Autodesk Inventor part; units mm, degrees
ref_plane "Work Plane1" through (0, 0, 0) normal (0, -1, 0) x (1, 0, 0)
ref_plane "YZ Plane" through (0, 0, 0) normal (1, 0, 0) x (0, 1, 0)
ref_plane "XZ Plane" through (0, 0, 0) normal (0, 1, 0) x (-1, 0, 0)
sketch "Sketch1" plane through (0, 0, 0) normal (0, 1, 0) x (-1, 0, 0)
  line L0 (0, 0) -> (27, 0)
  line L1 (27, 0) -> (27, -24)
  line L2 (27, -24) -> (0, -24)
  line L3 (0, -24) -> (0, 0)
  dimension "d0" = 27
  dimension "d1" = 24
extrude "Extrusion1" add sketch "Sketch1" along normal blind 8
sketch "Sketch2" plane through (0, 0, -24) normal (0, 0, -1) x (-1, 0, 0)
  line L0 (0, 0) -> (27, 0)
  line L1 (0, 0) -> (46.1678, 13.2384)
  line L2 (0, 0) -> (48.0283, 0) construction
  line L3 (0, 8) -> (27, 8)
  line L4 (27, 0) -> (27, 8)
  line L5 (0, 8) -> (27, 8)
  line L6 (27, 8) -> (27, 0)
  line L7 (27, 0) -> (0, 0)
  line L8 (0, 0) -> (0, 8)
  point P0 (27, 7.7421)
  dimension "d4" = 16
extrude "Extrusion2" cut sketch "Sketch2" against normal blind 30 contours L1 L4 L0
ref_plane "Work Plane1" through (0, 0, 0) normal (0, -1, 0) x (1, 0, 0)
sketch "Sketch3" plane through (0, 0, 0) normal (0, -1, 0) x (1, 0, 0)
  line L0 (0, 0) -> (0, -24)
  line L1 (0, -12) -> (-4, -12)
  circle A0 centre (-4, -12) radius 2.85
  line L2 (-4, -12) -> (-20, -12)
  line L3 (-12, -12) -> (-12, -20)
  line L4 (-12, -20) -> (-12, -4)
  circle A1 centre (-12, -20) radius 2.85
  circle A2 centre (-20, -12) radius 2.85
  circle A3 centre (-12, -4) radius 2.85
  dimension "d8" = 4
  dimension "d9" = 5.7
  dimension "d10" = 16
  dimension "d11" = 8
  dimension "d12" = 16
  dimension "d13" = 5.7
  dimension "d14" = 5.7
  dimension "d15" = 5.7
extrude "Extrusion3" add sketch "Sketch3" against normal blind 8
sketch "Sketch4" plane through (-4, 0, -12) normal (0, -1, 0) x (1, 0, 0)
  line L0 (4, 12) -> (4, -12)
  line L1 (4, -12) -> (-23.2805, -12)
  line L2 (-23.2805, -12) -> (-23.2805, 12)
  line L3 (-23.2805, 12) -> (4, 12)
  line L4 (4, 12) -> (4, -12)
extrude "Extrusion4" cut sketch "Sketch4" against normal blind 0.5
sketch "Sketch5" plane through (0, 8, 0) normal (0, 1, 0) x (1, 0, 0)
  line L0 (0, 0) -> (0, 24)
  line L1 (-27, 24) -> (-27, 0)
  line L2 (0, 0) -> (-27, 0)
  line L3 (-27, 0) -> (-27, 24)
  line L4 (-27, 24) -> (0, 24)
  line L5 (0, 24) -> (0, 0)
  circle A0 centre (-12, 4) radius 2.85
  circle A1 centre (-12, 20) radius 2.85
  line L6 (-12, 4) -> (-12, 20)
  arc A2 (-1.7437, 13.7412) -> (-1.7437, 10.2588) centre (-4, 12) ccw
  circle A3 centre (-20, 12) radius 2.85
  line L7 (-4, 12) -> (-20, 12)
  circle A4 centre (-12, 12) radius 1.65
  dimension "d20" = 3.3
extrude "Extrusion5" cut sketch "Sketch5" against normal blind 30 contours A4 L7 L6 | L6 L7 A4 | L7 A4 L6 | L6 A4 L7
sketch "Sketch6" plane through (0, 8, 0) normal (0, 1, 0) x (1, 0, 0)
  circle A0 centre (-12, 12) radius 1.65
  circle A1 centre (-12, 12) radius 2.9
  point P0 (0, 0)
  dimension "d23" = 5.8
extrude "Extrusion6" cut sketch "Sketch6" against normal blind 2
sketch "Sketch7" plane through (0, 8, 0) normal (0, 1, 0) x (1, 0, 0)
  line L0 (0, 24) -> (-27, 24)
  line L1 (0, 0) -> (-27, 0)
  line L2 (-27, 0) -> (-27, 24)
  line L3 (-27, 24) -> (0, 24)
  line L4 (0, 24) -> (0, 0)
  circle A0 centre (-12, 12) radius 1.65
  circle A1 centre (-12, 12) radius 2.9
extrude "Extrusion7" add sketch "Sketch7" along normal blind 4 contours L4 L1 L2 L0
sketch "Sketch8" plane through (0, 12, 0) normal (0, 1, 0) x (1, 0, 0)
  circle A0 centre (-12, 12) radius 2.9
  line L0 (-12, 12) -> (-12, -7.1279)
  line L1 (-27, 0) -> (0, 0)
  line L2 (-12, 12) -> (3.3617, 12)
  line L3 (3.3617, 12) -> (3.3617, -5.9927)
  line L4 (3.3617, -5.9927) -> (-12, -5.9927)
  line L5 (-12, -5.9927) -> (-12, 12)
  line L6 (-12, 12) -> (-14, 12)
  line L7 (-14, 12) -> (-14, -1.5388)
  line L8 (-12, 12) -> (-12, 14)
  line L9 (-12, 14) -> (5.1891, 14)
  line L10 (-14, -1.5388) -> (5.1891, -1.5388)
  line L11 (5.1891, -1.5388) -> (5.1891, 14)
  line L12 (5.1891, 14) -> (-14, 14)
  line L13 (-14, 14) -> (-14, -1.5388)
  point P0 (-14, 9.9)
  point P1 (-14, 0)
  point P2 (-12, 0)
  point P3 (-12, -1.5388)
  point P4 (-9.9, 14)
  dimension "d28" = 2
  dimension "d29" = 2
extrude "Extrusion8" cut sketch "Sketch8" against normal blind 4 contours L2 L3 L10 L0 A0 | A0 L9 L11 L10 L3 L2 | L0 L1 L7 A0
sketch "Sketch10" plane through (0, 12, 0) normal (0, 1, 0) x (1, 0, 0)
  line L0 (0, 14) -> (0, 0)
  line L1 (-27, 24) -> (-27, 0)
  line L2 (0, 0) -> (-27, 0)
  line L3 (-27, 0) -> (-27, 24)
  line L4 (-27, 24) -> (0, 24)
  line L5 (0, 24) -> (0, 0)
extrude "Extrusion10" cut sketch "Sketch10" against normal blind 4
sketch "Sketch11" plane through (0, 8, 0) normal (0, 1, 0) x (1, 0, 0)
  line L0 (-1.7437, 24) -> (-27, 24)
  line L1 (-27, 24) -> (0, 24)
  line L2 (0, 24) -> (-13.5, 24)
  line L3 (-13.5, 24) -> (-13.5, 22)
  line L4 (-27, 0) -> (-1.7437, 0)
  line L5 (-27, 0) -> (0, 0)
  circle A0 centre (-12, 12) radius 1.65
  line L6 (-12, 12) -> (-12, -4.3562)
  line L7 (-12, -4.3562) -> (-12, 27.2097)
  line L8 (-1.7437, 0) -> (0, 0)
  line L9 (-27, 24) -> (-27, 0)
  line L10 (0, 0) -> (-27, 0)
  line L11 (-27, 0) -> (-27, 24)
  line L12 (-27, 24) -> (0, 24)
  line L13 (0, 24) -> (0, 0)
  line L14 (-12, 0) -> (-12, 2)
  line L15 (-12, 24) -> (-12, 22)
  circle A1 centre (-12, 22) radius 1
  circle A2 centre (-12, 2) radius 1
  dimension "d36" = 2
  dimension "d37" = 2
  dimension "d38" = 2
  dimension "d39" = 2
  dimension "d40" = 2
extrude "Extrusion11" cut sketch "Sketch11" against normal blind 3 contours A1 L7 | L7 A1 | A2 L6 | L6 A2
properties part number "aruco_attachment_v1"
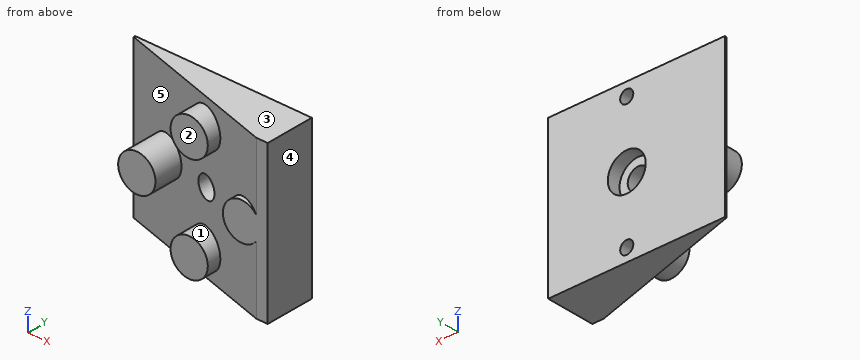
Could you check a few things on this model? Use its own coordinates, in mm. Face numbers are marked on the shaded views. A direction names the side the tool comes from. Coordinates: 2 decimals unless noted, no trailing zeros. Write each loop counter-clockwise with the first axis right and the second up, starting at its lowest first coordinate (ties: lowest second). Pieces come first, ordered by that corner, then holes. Notation, with made-up numbers: (22, 52.25) - (72, 52.25) arc R21 cw to (72, 62.25) - close; hole circle Ø2 at (17.5, -32.5). An arc over 180 degrees is marked (long way). Use a Markdown table: item, result.
Q1. Please list where these lines run through material, in increasing order: L1, parallel to Z at x = -12, y = 7.2; L2, parallel to Z at x = -12, y = 4.7; L3, parallel to Z at x = -10, y = 1.
Geometry check:
| item | result |
|---|---|
| L1 | z = -24 to -23, -21 to -14.9, -9.1 to -3, -1 to 0 |
| L2 | z = -24 to -13.65, -10.35 to 0 |
| L3 | z = -22.03 to -17.97, -6.03 to -1.97 |
Q2. Thinking about a two-plate mould opening in Z: for the marked faces 1, 2 and 3, which applies, +Z half, -Z half, draft (parallel to the pull), parting line (faces both ways), or undercut?
Geometry check:
| item | result |
|---|---|
| face 1 | undercut |
| face 2 | draft |
| face 3 | +Z half |
Q3. Imagine slicing it at C-C (x = -20). List the corners of the cut face in (y, z) for me.
Geometry check:
| item | result |
|---|---|
| outline | (0.5, -14.85) - (5.73, -14.85) - (5.73, -24) - (8, -24) - (8, 0) - (5.73, 0) - (5.73, -9.15) - (0.5, -9.15) - close |
Q4. Imagine slicing it at B-B (y = 7). List the corners of the cut face in (x, z) for me, and give its area (3 significant figures).
Geometry check:
| item | result |
|---|---|
| outline | (-24.41, -24) - (0, -24) - (0, 0) - (-24.41, 0) - close; hole circle Ø5.8 at (-12, -12); hole circle Ø2 at (-12, -22); hole circle Ø2 at (-12, -2) |
| area | 553 mm2 |
Q5. Which directions (+Z, -Z, +X, -X, +Y, -Y) give clear straight access to the entire face, cutting with the end or side of a thin tool? Please do the marked faces 4 and 5.
Geometry check:
| item | result |
|---|---|
| face 4 | +Z, -Z, +X, +Y, -Y |
| face 5 | -Y |
Q6. I'm going to push flat-ended pins straight in: pin 1 Ø0.6 at (x, z) = (-12, -21.5) entering from +Y; pin 2 Ø5 at (x, z) = (-12, -12) entering from +Y; pin 3 Ø4 at (y, z) = (7, -11) entering from -X; pin 4 Ø2.5 at (x, z) = (-12, -12) entering from +Y. Where does each tip first touch, or does it pass through?
Geometry check:
| item | result |
|---|---|
| pin 1 | stops at y = 5 |
| pin 2 | stops at y = 6 |
| pin 3 | stops at x = -27 |
| pin 4 | passes through |
Q7. Imagine slicing it at A-A (z = -12). List the corners of the cut face in (x, y) for me, and give its area (3 significant figures).
Geometry check:
| item | result |
|---|---|
| outline | (-27, 7.74) - (-22.85, 6.55) - (-22.85, 0.5) - (-17.15, 0.5) - (-17.15, 4.92) - (-13.65, 3.91) - (-13.65, 6) - (-14.9, 6) - (-14.9, 8) - (-27, 8) - close; (-10.35, 2.97) - (-6.85, 1.96) - (-6.85, 0.5) - (0, 0.5) - (0, 8) - (-9.1, 8) - (-9.1, 6) - (-10.35, 6) - close |
| area | 125 mm2 |
Q8. Imagine slicing it at D-D (z = -20). List the corners of the cut face in (x, y) for me, and give its area (3 significant figures).
Geometry check:
| item | result |
|---|---|
| outline | (-27, 7.74) - (-14.85, 4.26) - (-14.85, 0.5) - (-9.15, 0.5) - (-9.15, 2.62) - (-1.74, 0.5) - (0, 0.5) - (0, 8) - (-27, 8) - close |
| area | 128 mm2 |
